Here's how the part is built. I have some questions about the finished solid (model axes, mm). A direction names the side the tool comes from. Give positions to 0.01 mm unless a question says otherwise; leave off trailing zeros. Loops run counter-clockwise (first coordinate to the right, second up) from the corner with the lowest first, then second, coordinate; pieces in that order, holes last. Notation, with made-up numbers: (-34, 9.5) - (23, 9.5) arc R31 cw to (23, 48.5) - close; hole circle Ø11 at (55, 63). An arc over 180 degrees is marked (long way). Use one line per item in the form item = value.
from build123d import *

# Parameters (mm, degrees)
F1_DEPTH = 19.05
F2_R     = 44.45
F3_DEPTH = 101.6
F4_W     = 254
F4_H     = 50.8
F5_DEPTH = 127
F7_DEPTH = 88.9
F8_R     = 50.8
F9_DEPTH = 19.051


with BuildPart() as f1:
    # F0 (on Front) → F1 (new body)
    with BuildSketch(Plane.XZ):
        with BuildLine():
            Line((0, 50.8), (0, 0))
            Line((0, 0), (254, 0))
            Line((254, 0), (254, 50.8))
            Line((254, 50.8), (186.227747, 226.098122))
            ThreePointArc((186.227747, 226.098122), (127, 266.7), (67.772253, 226.098122))
            Line((67.772253, 226.098122), (0, 50.8))
        make_face()
    extrude(amount=F1_DEPTH)

    # F2 (on face) → F3 (join)
    with BuildSketch(Plane.XZ.offset(19.05)):
        with BuildLine():
            ThreePointArc((67.772253, 226.098122), (115.353368, 140.7772), (190.5, 203.2))
            ThreePointArc((190.5, 203.2), (189.4228, 214.846632), (186.227747, 226.098122))
            ThreePointArc((186.227747, 226.098122), (127, 266.7), (67.772253, 226.098122))
        make_face()
        with Locations((127, 203.2)):
            Circle(F2_R, mode=Mode.SUBTRACT)
    extrude(amount=F3_DEPTH)

    # F4 (on face) → F5 (join)
    with BuildSketch(Plane.XZ.offset(19.05)):
        with Locations((127, 25.4)):
            Rectangle(F4_W, F4_H)
    extrude(amount=F5_DEPTH)

    # F6 (on face) → F7 (join)
    with BuildSketch(Plane.XZ.offset(19.05)):
        with BuildLine():
            Line((117.475, 140.418439), (117.475, 50.8))
            Line((117.475, 50.8), (136.525, 50.8))
            Line((136.525, 50.8), (136.525, 140.418439))
            ThreePointArc((136.525, 140.418439), (127, 139.820783), (117.475, 140.418439))
        make_face()
    extrude(amount=F7_DEPTH)

    # F8 (on face) → F9 (cut, through all)
    with BuildSketch(Plane.XZ.offset(19.05)):
        with Locations((127, 203.2)):
            Circle(F8_R)
    extrude(amount=-F9_DEPTH, mode=Mode.SUBTRACT)


solid = f1.part
(1) If we section it at B-B (x = 127): List the corners of the cut face in (y, z) for me, plus the area to 3 significant figures.
Geometry says:
outline = (-146.05, 0) - (0, 0) - (0, 152.4) - (-19.05, 152.4) - (-19.05, 158.75) - (-120.65, 158.75) - (-120.65, 139.7) - (-107.95, 139.7) - (-107.95, 50.8) - (-146.05, 50.8) - close; (-120.65, 247.65) - (-19.05, 247.65) - (-19.05, 254) - (0, 254) - (0, 266.7) - (-120.65, 266.7) - close
area = 21,400 mm²
(2) If we section it at C-C (z = 72): List the corners of the cut face in (x, y) for me (3 decimals).
Geometry says:
outline = (8.196, -19.05) - (117.475, -19.05) - (117.475, -107.95) - (136.525, -107.95) - (136.525, -19.05) - (245.804, -19.05) - (245.804, 0) - (8.196, 0) - close
(3) If I drill on probe 1 along Z at (x, y) = (127, -61); probe 2 along X at (y, z) = (-87, 203); probe 3 along Y at (x, z) = (201, 92.5), over which ranges is the centre line in solid material (lowest first)?
Geometry says:
probe_1 = 0 to 158.75, 247.65 to 266.7
probe_2 = 63.5 to 82.55, 171.45 to 190.5
probe_3 = -19.05 to 0
(4) Thinking about a two-plate mould opening in X: for faces 5 (the flat face through (125, 0, 106)), 6 (the flat face through (127, -19.05, 158)), 7 (the flat face through (254, -72, 25)), 8 (the flat face through (117.475, -63, 96)), which applies, pulls with the +X half, pulls with the -X half, needs draft (parallel to the pull), parting line crosses it, or undercut?
Geometry says:
face_5 = needs draft
face_6 = undercut
face_7 = pulls with the +X half
face_8 = pulls with the -X half
(5) For P1, Ø3, axis at x = 117, z = 101.5, coming from the -Y side; P2, Ø12, axis at y = -119.5, z = 202, coming from the +X side; P3, Ø8, axis at x = 134, y = -105, coming from the +Z side, each with a flat end and sliding along its axis, tell me the tip position at first contact or that it passes through.
Geometry says:
P1 = -107.95
P2 = 190.5
P3 = 266.63
(6) If we section it at A-A (y = -83): List the corners of the cut face in (x, z) for me (3 decimals), plus the area to 3 significant figures.
Geometry says:
outline = (0, 0) - (254, 0) - (254, 50.8) - (136.525, 50.8) - (136.525, 140.418) arc R63.5 ccw to (190.5, 203.2) arc R63.5 ccw to (186.228, 226.098) arc R63.5 ccw (long way) to (117.475, 140.418) - (117.475, 50.8) - (0, 50.8) - close; hole circle Ø88.9 at (127, 203.2)
area = 21,100 mm²
(7) For faces 1 (the flat face through (71, -19.05, 101)), 2 (the flat face through (125, -110, 50.8)), 3 (the flat face through (140, -120.65, 246)), 4 (the cylindrical face through (150.44, -9.66, 158.13)), which set-ups out of +Z, -Z, +X, -X, +Y, -Y let a thin tool reach every point of the face, with its end or its side?
Geometry says:
face_1 = -X, -Y
face_2 = -Y
face_3 = +Z, +X, -X, -Y
face_4 = +Y
(8) If we section it at D-D (z = 173): List the corners of the cut face in (x, y) for me, plus the area to 3 significant figures.
Geometry says:
outline = (47.24, -19.05) - (71.14, -19.05) - (71.14, -120.65) - (94.38, -120.65) - (94.38, -19.05) - (86.15, -19.05) - (86.15, 0) - (47.24, 0) - close; (159.62, -120.65) - (182.86, -120.65) - (182.86, -19.05) - (206.76, -19.05) - (206.76, 0) - (167.85, 0) - (167.85, -19.05) - (159.62, -19.05) - close
area = 6,210 mm²
